from build123d import *

# Parameters (mm, degrees)
SKETCH2_R          = 1.25
CUT_EXTRUDE1_DEPTH = 19.25
FILLET1_R          = 2
SKETCH3_R          = 2.5
CUT_EXTRUDE2_DEPTH = 13.25
SKETCH4_R          = 11
CUT_EXTRUDE3_DEPTH = 6


with BuildPart() as part:
    # Sketch1 → Revolve1 (revolve)
    with BuildSketch(Plane(origin=(0, 0, 0), x_dir=(1, 0, 0), z_dir=(0, 1, 0))):
        Polygon((-6.130434783, 14.45), (6.626387667, 14.45), (10.619565217, 11.440924884), (10.619565217, 4), (14.619565217, 4), (14.619565217, 0), (13.372742768, 0), (-6.130434783, 0), (-7.630434783, 0), (-7.630434783, 18.25), (-6.130434783, 18.25), align=None)
    revolve(axis=Axis((-12.391304348, 0, 0), (1, 0, 0)))

    # Sketch2 → Cut-Extrude1 (cut, through all)
    with BuildSketch(Plane(origin=(10.619565217, 0, 0), x_dir=(0, 0, -1), z_dir=(1, 0, 0))):
        with Locations((0, 9.5)):
            Circle(SKETCH2_R)
        with Locations((6.717514421, 6.717514421)):
            Circle(SKETCH2_R)
        with Locations((9.5, 0)):
            Circle(SKETCH2_R)
        with Locations((6.717514421, -6.717514421)):
            Circle(SKETCH2_R)
        with Locations((0, -9.5)):
            Circle(SKETCH2_R)
        with Locations((-6.717514421, -6.717514421)):
            Circle(SKETCH2_R)
        with Locations((-9.5, 0)):
            Circle(SKETCH2_R)
        with Locations((-6.717514421, 6.717514421)):
            Circle(SKETCH2_R)
    extrude(amount=-CUT_EXTRUDE1_DEPTH, mode=Mode.SUBTRACT)

    # Fillet1
    fillet1_edges = [part.edges().sort_by_distance(p)[0] for p in [
        (14.619565217, 0, 4),
    ]]
    fillet(fillet1_edges, radius=FILLET1_R)

    # Sketch3 → Cut-Extrude2 (cut)
    with BuildSketch(Plane.ZY.offset(7.630434783)):
        with Locations((0, 9.5)):
            Circle(SKETCH3_R)
        with Locations((6.717514421, 6.717514421)):
            Circle(SKETCH3_R)
        with Locations((9.5, 0)):
            Circle(SKETCH3_R)
        with Locations((6.717514421, -6.717514421)):
            Circle(SKETCH3_R)
        with Locations((0, -9.5)):
            Circle(SKETCH3_R)
        with Locations((-6.717514421, -6.717514421)):
            Circle(SKETCH3_R)
        with Locations((-9.5, 0)):
            Circle(SKETCH3_R)
        with Locations((-6.717514421, 6.717514421)):
            Circle(SKETCH3_R)
    extrude(amount=-CUT_EXTRUDE2_DEPTH, mode=Mode.SUBTRACT)

    # Sketch4 → Cut-Extrude3 (cut)
    with BuildSketch(Plane.ZY.offset(7.630434783)):
        Circle(SKETCH4_R)
    extrude(amount=-CUT_EXTRUDE3_DEPTH, mode=Mode.SUBTRACT)


solid = part.part
Here's how the part is built. I have some questions about the finished solid (model axes, mm). A direction names the side the tool comes from. Round coordinates to 2 decimals unless told otherwise and drop trailing zeros. Loops run counter-clockwise (first coordinate to the right, second up) from the corner with the lowest first, then second, coordinate; pieces in that order, holes last.
1. We'd pull the mould along Z, two halves only. Please class faces 3 (the face through (-6.87, -17.816, 3.956)), 4 (the face through (-6.13, 10, 11)), 5 (the face through (8.15, 10.74, 0.16)): +Z half, -Z half, draft (parallel to the pull), parting line (faces both ways), or undercut.
Answer list:
face 3: parting line
face 4: draft
face 5: undercut
2. If we section it at A-A on x = -5.5: Write out the boundary of the cut face in (y, z).
Answer list:
outline: circle Ø28.9 at (0, 0); hole (-10.79, -2.14) arc R11 ccw to (-9.14, -6.11) arc R2.5 ccw to (-6.11, -9.14) arc R11 ccw to (-2.14, -10.79) arc R2.5 ccw to (2.14, -10.79) arc R11 ccw to (6.11, -9.14) arc R2.5 ccw to (9.14, -6.11) arc R11 ccw to (10.79, -2.14) arc R2.5 ccw to (10.79, 2.14) arc R11 ccw to (9.14, 6.11) arc R2.5 ccw to (6.11, 9.14) arc R11 ccw to (2.14, 10.79) arc R2.5 ccw to (-2.14, 10.79) arc R11 ccw to (-6.11, 9.14) arc R2.5 ccw to (-9.14, 6.11) arc R11 ccw to (-10.79, 2.14) arc R2.5 ccw to start
3. For P1, Ø4, axis at y = 9, z = -0.5, coming from the -X side; P2, Ø5, axis at x = -1.5, y = -8, coming from the -Z side; P3, Ø6, axis at y = -6.72, z = 6.72, coming from the -X side; P4, Ø1.5, axis at y = -6.5, z = -7.5, coming from the -X side, each with a flat end and sliding along its axis, tell me the tip position at first contact or that it passes through.
Answer list:
P1: stops at x = -1.63
P2: stops at z = -13.36
P3: stops at x = -7.63
P4: stops at x = 5.62
4. Which directions (+Z, -Z, +X, -X, +Y, -Y) give clear straight access to the entire face, cutting with the end or side of a thin tool? Please do faces 1 (the face through (5.62, -6, -8)), 2 (the face through (8.155, 6.772, 7.966)).
Answer list:
face 1: -X
face 2: +X, -X
5. If I drill on line 1 along Y through (x, z) = (-6.25, 0); line 2 along Y through (x, z) = (7.8, 0); line 3 along Y through (x, z) = (1.75, 0), over which ranges is the centre line in solid material (lowest first)?
Answer list:
line 1: y = -18.25 to -12, 12 to 18.25
line 2: y = -13.57 to -10.75, -8.25 to 8.25, 10.75 to 13.57
line 3: y = -14.45 to -12, -7 to 7, 12 to 14.45
6. If we section it at B-B on y = 0: Count the separate pieces of the cut face and the enclosed holes in it, plus the area to 3 significant figures.
Answer list:
separate pieces: 3
enclosed holes: 0
area: 316 mm2
